Read the model definition and answer for the solid it produces. Units are mm, in the model's axes. A direction names the side the tool comes from. Give positions to 0.01 mm unless a question says otherwise; leave off trailing zeros. Order: outer loops, then holes, each group sorted by start corner. A loop starts at its lowest first (then second) coordinate and runs counter-clockwise, first axis right, second up. Notation, with made-up numbers: (-6, 46) - (49, 46) arc R30 cw to (49, 76) - close; hole circle Ø3 at (28.25, 26.5). An arc over 180 degrees is marked (long way). Write each question's results on one line, items separated by ' | '.
from build123d import *

# Parameters (mm, degrees)
BOSS_EXTRUDE1_DEPTH     = 65.33
CHAMFER1_SIZE           = 5.8
BOSS_EXTRUDE2_DEPTH     = 2.52
BOSS_EXTRUDE3_DEPTH     = 2.52
SKETCH4_R               = 19.03
SKETCH4_R_2             = 2.58
CUT_EXTRUDE1_DEPTH      = 4.1
CUT_EXTRUDE2_DEPTH      = 66.7
CUT_EXTRUDE2_DEPTH_BACK = 4.1


with BuildPart() as part:
    # Sketch1 → Boss-Extrude1 (new body)
    with BuildSketch(Plane(origin=(0, 0, 0), x_dir=(0, 0, -1), z_dir=(1, 0, 0))):
        with BuildLine():
            Line((0, 0), (0, 64.22))
            Line((0, 64.22), (-3.1, 64.22))
            Line((-3.1, 64.22), (-3.1, 0))
            ThreePointArc((-3.1, 0), (-1.758549058, -3.238549058), (1.48, -4.58))
            Line((1.48, -4.58), (65.7, -4.58))
            Line((65.7, -4.58), (65.7, -1.48))
            Line((65.7, -1.48), (1.48, -1.48))
            ThreePointArc((1.48, -1.48), (0.433481964, -1.046518036), (0, 0))
        make_face()
    extrude(amount=BOSS_EXTRUDE1_DEPTH)

    # Chamfer1
    chamfer1_edges = [part.edges().sort_by_distance(p)[0] for p in [
        (65.33, 64.22, 1.55),
        (65.33, -3.03, -65.7),
        (0, -3.03, -65.7),
        (0, 64.22, 1.55),
    ]]
    chamfer(chamfer1_edges, length=CHAMFER1_SIZE)

    # Sketch2 → Boss-Extrude2 (add)
    with BuildSketch(Plane(origin=(65.33, 0, 0), x_dir=(0, 0, -1), z_dir=(1, 0, 0))):
        Polygon((0, 27.49), (17.41, -1.48), (0, -1.48), align=None)
    extrude(amount=-BOSS_EXTRUDE2_DEPTH)

    # Sketch3 → Boss-Extrude3 (add)
    with BuildSketch(Plane.ZY):
        Polygon((0, 27.49), (-17.41, -1.48), (0, -1.48), align=None)
    extrude(amount=-BOSS_EXTRUDE3_DEPTH)

    # Sketch4 → Cut-Extrude1 (cut, through all)
    with BuildSketch(Plane(origin=(0, 0, 0), x_dir=(-1, 0, 0), z_dir=(0, 0, -1))):
        with Locations((-32.665, 35.09)):
            Circle(SKETCH4_R)
        with Locations((-56.235, 58.66)):
            Circle(SKETCH4_R_2)
        with Locations((-9.095, 58.66)):
            Circle(SKETCH4_R_2)
        with Locations((-9.095, 11.52)):
            Circle(SKETCH4_R_2)
        with Locations((-56.235, 11.52)):
            Circle(SKETCH4_R_2)
    extrude(amount=-CUT_EXTRUDE1_DEPTH, mode=Mode.SUBTRACT)

    # Sketch5 → Cut-Extrude2 (cut, two sides)
    with BuildSketch(Plane(origin=(0, -1.48, 0), x_dir=(1, 0, 0), z_dir=(0, 1, 0))) as cut_extrude2_sk:
        with BuildLine():
            Line((50.635, 9.67), (50.635, 59.84))
            ThreePointArc((50.635, 59.84), (52.705, 61.91), (54.775, 59.84))
            Line((54.775, 59.84), (54.775, 9.67))
            ThreePointArc((54.775, 9.67), (52.705, 7.6), (50.635, 9.67))
        make_face()
        with BuildLine():
            Line((10.555, 9.67), (10.555, 59.84))
            ThreePointArc((10.555, 59.84), (12.625, 61.91), (14.695, 59.84))
            Line((14.695, 59.84), (14.695, 9.67))
            ThreePointArc((14.695, 9.67), (12.625, 7.6), (10.555, 9.67))
        make_face()
    extrude(amount=CUT_EXTRUDE2_DEPTH, mode=Mode.SUBTRACT)
    extrude(cut_extrude2_sk.sketch, amount=-CUT_EXTRUDE2_DEPTH_BACK, mode=Mode.SUBTRACT)


solid = part.part
(1) Section D-D (x = 4.5) is taken. Give the vertices of the cut face in (y, z), plus the area to 3 significant figures.
Conclusion:
outline: (-4.58, -64.4) - (-1.48, -64.4) - (-1.48, -1.48) arc R1.48 cw to (0, 0) - (62.92, 0) - (62.92, 3.1) - (0, 3.1) arc R4.58 ccw to (-4.58, -1.48) - close | area: 405 mm^2
(2) Section C-C (x = 25.5) is taken. Give the vertices of the cut face in (y, z).
Conclusion:
outline: (-4.58, -65.7) - (-1.48, -65.7) - (-1.48, -1.48) arc R1.48 cw to (0, 0) - (17.46, 0) - (17.46, 3.1) - (0, 3.1) arc R4.58 ccw to (-4.58, -1.48) - close; (52.72, 0) - (64.22, 0) - (64.22, 3.1) - (52.72, 3.1) - close
(3) Consider probe 1 along X at (y, z) = (11, 2); probe 2 along Z at (x, y) = (58, 25.5); probe 3 along Y at (x, z) = (16, -11). Determine where each line is inside the solid, lowest interval first. Write a range as [from, to].
Conclusion:
probe 1: [0, 6.57], [11.62, 53.71], [58.76, 65.33] | probe 2: [0, 3.1] | probe 3: [-4.58, -1.48]
(4) For faces 4 (the face through (2.52, 7, -5)), 5 (the face through (32, -3, -65.7)), 6 (the face through (54.775, -3, -35)), determine the directions among +Z, -Z, +X, -X, +Y, -Y from which every point of the face is accessible in a straight line to the end or side of a thin tool.
Conclusion:
face 4: -Z, +Y | face 5: -Z, +X, -X, +Y, -Y | face 6: +Y, -Y
(5) Each of these flat-tipped pins is pushed along its axis until it touches: pin 1 (8.5 mm diameter, centred on x = 56.235, y = 11.52, fed in from -Z); pin 2 (4 mm diameter, centred on x = 9.095, y = 58.66, fed in from +Z); pin 3 (19.5 mm diameter, centred on x = 21, z = -28, fed in from +Y). Where does it stop, or does it pass through?
Conclusion:
pin 1: z = 0 | pin 2: through | pin 3: y = -1.48
(6) Section B-B (z = -55.5) is taken. Give the vertices of the cut face in (x, y) (3 decimals).
Conclusion:
outline: (0, -4.58) - (10.555, -4.58) - (10.555, -1.48) - (0, -1.48) - close; (14.695, -4.58) - (50.635, -4.58) - (50.635, -1.48) - (14.695, -1.48) - close; (54.775, -4.58) - (65.33, -4.58) - (65.33, -1.48) - (54.775, -1.48) - close
(7) The mould has two halves that part along Z. Classify faces 1 (the face through (10.555, -3, -34)), 2 (the face through (32, -4.58, -33)), 3 (the face through (64.09, 13.21, -8.58)): pulls with the +Z half, pulls with the -Z half, needs draft (parallel to the pull), parting line crosses it, or undercut.
Conclusion:
face 1: undercut | face 2: needs draft | face 3: pulls with the -Z half
(8) Section A-A (y = 42.5) is taken. Give the vertices of the cut face in (x, z), plus the area to 3 significant figures.
Conclusion:
outline: (0, 0) - (15.14, 0) - (15.14, 3.1) - (0, 3.1) - close; (50.19, 0) - (65.33, 0) - (65.33, 3.1) - (50.19, 3.1) - close | area: 93.8 mm^2
